from build123d import *

# Parameters (mm, degrees)
ESQUISSE2_R             = 100
ESQUISSE2_W             = 60
ESQUISSE2_H             = 60
BOSS_EXTRU_6_DEPTH      = 20
ESQUISSE3_W             = 60
ESQUISSE3_H             = 30
ESQUISSE3_W_2           = 30
ESQUISSE3_H_2           = 60
ENL_V_MAT_EXTRU_7_DEPTH = 10
ESQUISSE7_R             = 2
ENL_V_MAT_EXTRU_8_DEPTH = 20


with BuildPart() as part:
    # Esquisse2 → Boss.-Extru.6 (new body)
    with BuildSketch(Plane(origin=(0, 0, 0), x_dir=(1, 0, 0), z_dir=(0, 1, 0))):
        with Locations(Location((0, 0, 0), (0, 0, 270))):
            Circle(ESQUISSE2_R)
        Rectangle(ESQUISSE2_W, ESQUISSE2_H, mode=Mode.SUBTRACT)
    extrude(amount=BOSS_EXTRU_6_DEPTH)

    # Esquisse3 → Enlèv. mat.-Extru.7 (cut)
    with BuildSketch(Plane(origin=(0, 20, 0), x_dir=(1, 0, 0), z_dir=(0, 1, 0))):
        with Locations((0, 45)):
            Rectangle(ESQUISSE3_W, ESQUISSE3_H)
        with Locations((45, 0)):
            Rectangle(ESQUISSE3_W_2, ESQUISSE3_H_2)
        with Locations((0, -45)):
            Rectangle(ESQUISSE3_W, ESQUISSE3_H)
        with Locations((-45, 0)):
            Rectangle(ESQUISSE3_W_2, ESQUISSE3_H_2)
    extrude(amount=-ENL_V_MAT_EXTRU_7_DEPTH, mode=Mode.SUBTRACT)

    # Esquisse7 → Enlèv. mat.-Extru.8 (cut)
    with BuildSketch(Plane(origin=(0, 20, 0), x_dir=(1, 0, 0), z_dir=(0, 1, 0))):
        with Locations(Location((0, 90, 0), (0, 0, 270))):
            Circle(ESQUISSE7_R)
        with Locations(Location((90, 0, 0), (0, 0, 270))):
            Circle(ESQUISSE7_R)
        with Locations(Location((0, -90, 0), (0, 0, 270))):
            Circle(ESQUISSE7_R)
        with Locations(Location((-90, 0, 0), (0, 0, 270))):
            Circle(ESQUISSE7_R)
    extrude(amount=-ENL_V_MAT_EXTRU_8_DEPTH, mode=Mode.SUBTRACT)


solid = part.part
The listing builds one solid part. Answer for the finished solid, in the listing's coordinates (mm). A direction names the side the tool comes from. Coordinates: 2 decimals unless noted, no trailing zeros. Loops run counter-clockwise (first coordinate to the right, second up) from the corner with the lowest first, then second, coordinate; pieces in that order, holes last.
1) Flat-ended cylindrical pins translate along their axes: pin 1 Ø6 at (y, z) = (2.5, -70) entering from -X; pin 2 Ø11 at (x, y) = (-50, 16.5) entering from +Z; pin 3 Ø24 at (x, z) = (11, -47) entering from +Y. Find the tip coordinate at first contact, or state that the pin passes through.
2) Determine the mould class of faces 3 (the face through (30.04, 9.86, 95.38)), 4 (the face through (-30, 15, 45)), 5 (the face through (-60, 15, 0)), 6 (the face through (-43, 20, 43)) for opening direction X: pulls with the +X half, pulls with the -X half, needs draft (parallel to the pull), parting line crosses it, or undercut.
3) Find section D-D on z = 36.5. Write down the section's boundary in (x, y), then the cut area to 3 significant figures.
4) Find section B-B on z = 4.5. Write down the section's boundary in (x, y), then the cut area to 3 significant figures.
5) Find the intervals of material crossed by L1, parallel to X at y = 9, z = 0; L2, parallel to X at y = 14.5, z = -22; L3, parallel to Z at x = 32, y = 15.75, in increasing order.
6) Find section A-A on y = 5. Write down the section's boundary in (x, z), then the cut area to 3 significant figures.
7) Find section C-C on x = -20. Write down the section's boundary in (y, z).
8) A tool of negligible diameter and unlimited length cuts with its end or side. For faces 1 (the face through (0, 5, 30)), 2 (the face through (30, 15, -45)), from which of +Z, -Z, +X, -X, +Y, -Y can it reach the whole face along a straight path? Write none if from no direction.
Values:
1. pin 1: stops at x = -74.24
1. pin 2: stops at z = 89.55
1. pin 3: stops at y = 10
2. face 3: parting line crosses it
2. face 4: undercut
2. face 5: undercut
2. face 6: needs draft
3. outline: (-93.1, 0) - (93.1, 0) - (93.1, 20) - (30, 20) - (30, 10) - (-30, 10) - (-30, 20) - (-93.1, 20) - close
3. area: 3,120 mm2
4. outline: (-99.9, 0) - (-30, 0) - (-30, 10) - (-60, 10) - (-60, 20) - (-99.9, 20) - close; (30, 0) - (99.9, 0) - (99.9, 20) - (60, 20) - (60, 10) - (30, 10) - close
4. area: 2,200 mm2
5. L1: x = -100 to -92, -88 to -30, 30 to 88, 92 to 100
5. L2: x = -97.55 to -60, 60 to 97.55
5. L3: z = -94.74 to -30, 30 to 94.74
6. outline: circle Ø200 at (0, 0); hole circle Ø4 at (-90, 0); hole (-30, -30) - (30, -30) - (30, 30) - (-30, 30) - close; hole circle Ø4 at (0, -90); hole circle Ø4 at (0, 90); hole circle Ø4 at (90, 0)
6. area: 27,800 mm2
7. outline: (0, -97.98) - (20, -97.98) - (20, -60) - (10, -60) - (10, -30) - (0, -30) - close; (0, 30) - (10, 30) - (10, 60) - (20, 60) - (20, 97.98) - (0, 97.98) - close
8. face 1: +Y, -Y
8. face 2: +Y
